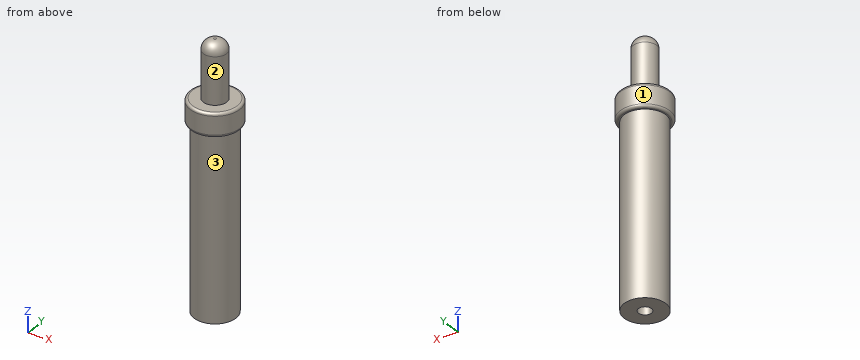
```python
from build123d import *

# Parameters (mm, degrees)
ESBO_O1_R                     = 4.7625
RESSALTO_EXTRUS_O1_DEPTH      = 50.5
FURO_ROSCADO_DE_M3X0_52_D     = 2.5
FURO_ROSCADO_DE_M3X0_52_DEPTH = 8.5
FURO_ROSCADO_DE_M3X0_52_TIP   = 0.751075774
ESBO_O8_OUTSIDE_W             = 21.979
ESBO_O8_OUTSIDE_H             = 21.979
ESBO_O8_OUTSIDE_R             = 4
CORTE_EXTRUS_O1_DEPTH         = 35
ESBO_O10_OUTSIDE_W            = 21.979
ESBO_O10_OUTSIDE_H            = 21.979
ESBO_O10_OUTSIDE_R            = 2.25
CORTE_EXTRUS_O2_DEPTH         = 11
FILETE1_R                     = 0.5
FILETE2_R                     = 2


with BuildPart() as part:
    # Esboço1 → Ressalto-extrusão1 (new body)
    with BuildSketch(Plane.XY):
        with Locations((240.708388302, 2.596082859)):
            Circle(ESBO_O1_R)
    extrude(amount=RESSALTO_EXTRUS_O1_DEPTH)

    # Furo roscado de M3x0.52
    with Locations(Plane(origin=(0, 0, 0), x_dir=(-1, 0, 0), z_dir=(0, 0, -1))):
        with Locations((-240.708388302, 2.596082859)):
            Hole(FURO_ROSCADO_DE_M3X0_52_D / 2, depth=FURO_ROSCADO_DE_M3X0_52_DEPTH)
            with Locations((0, 0, -(FURO_ROSCADO_DE_M3X0_52_DEPTH + FURO_ROSCADO_DE_M3X0_52_TIP / 2))):  # 118° drill point
                Cone(0, FURO_ROSCADO_DE_M3X0_52_D / 2, FURO_ROSCADO_DE_M3X0_52_TIP, mode=Mode.SUBTRACT)

    # Esboço8 outside → Corte-extrusão1 (cut)
    with BuildSketch(Plane(origin=(0, 0, 0), x_dir=(-1, 0, 0), z_dir=(0, 0, -1))):
        with Locations((-240.7085, 2.5965)):
            Rectangle(ESBO_O8_OUTSIDE_W, ESBO_O8_OUTSIDE_H)
        with Locations((-240.708388302, 2.596082859)):
            Circle(ESBO_O8_OUTSIDE_R, mode=Mode.SUBTRACT)
    extrude(amount=-CORTE_EXTRUS_O1_DEPTH, mode=Mode.SUBTRACT)

    # Esboço10 outside → Corte-extrusão2 (cut)
    with BuildSketch(Plane.XY.offset(50.5)):
        with Locations((240.7085, 2.5965)):
            Rectangle(ESBO_O10_OUTSIDE_W, ESBO_O10_OUTSIDE_H)
        with Locations((240.708388302, 2.596082859)):
            Circle(ESBO_O10_OUTSIDE_R, mode=Mode.SUBTRACT)
    extrude(amount=-CORTE_EXTRUS_O2_DEPTH, mode=Mode.SUBTRACT)

    # Filete1
    filete1_edges = [part.edges().sort_by_distance(p)[0] for p in [
        (235.945888302, 2.596082859, 35),
        (235.945888302, 2.596082859, 39.5),
    ]]
    fillet(filete1_edges, radius=FILETE1_R)

    # Filete2
    filete2_edges = [part.edges().sort_by_distance(p)[0] for p in [
        (238.458388302, 2.596082859, 50.5),
    ]]
    fillet(filete2_edges, radius=FILETE2_R)


solid = part.part
```
Geometry: final body of the model. Coordinates: model frame, mm. Face numbers are marked on the shaded views. A direction names the side the tool comes from. Coordinates: 2 decimals unless noted, no trailing zeros. Loops run counter-clockwise (first coordinate to the right, second up) from the corner with the lowest first, then second, coordinate; pieces in that order, holes last. Notation, with made-up numbers: (57, 48) -> (92, 48) arc R12 ccw to (92, 55) -> close; hole circle Ø10 at (70, 21.25). An arc over 180 degrees is marked (long way). Use a Markdown table: item, result. Add a question column.
(1) Pin query (flat end, axial travel): pin 1 Ø1 at (y, z) = (4.5, 27) entering from +X; pin 2 Ø3 at (y, z) = (1.5, 26) entering from -X; pin 3 Ø1 at (y, z) = (-1, 40.5) entering from +X; pin 4 Ø1.5 at (x, z) = (243, 23.5) entering from +Y. Return the tip coordinate at first contact, or that it passes through.
(2) Line query: line 1 along Z through (x, y) = (240, 5.5); line 2 along Y through (x, z) = (240.75, 9); line 3 along Z through (x, y) = (240.25, -1.5). Output: solid intervals per line, ascending.
(3) Access query for the marked faces 1, 2 and 3. Directions: +Z, -Z, +X, -X, +Y, -Y. A direction counts if a zero-diameter tool reaches every point of the face in a straight line with its end or side. Return the directions, or none.
(4) Section query A-A, the plane z = 8. Return loops of the section in (x, y).
(5) Section query B-B, the plane z = 47.5. Return loops of the section in (x, y), plus the area to 3 significant figures.
(6) Section query C-C, the plane z = 36. Return loops of the section in (x, y) (1 decimal).
Answer:
| question | item | result |
|---|---|---|
| 1 | pin 1 | stops at x = 244.45 |
| 1 | pin 2 | stops at x = 236.71 |
| 1 | pin 3 | passes through |
| 1 | pin 4 | stops at y = 6.29 |
| 2 | line 1 | z = 0 to 39.5 |
| 2 | line 2 | y = -1.4 to 2.18, 3.01 to 6.6 |
| 2 | line 3 | z = 35 to 39.5 |
| 3 | face 1 | +Z, -Z |
| 3 | face 2 | +Z |
| 3 | face 3 | -Z |
| 4 | outline | circle Ø8 at (240.71, 2.6); hole circle Ø2.5 at (240.71, 2.6) |
| 5 | outline | circle Ø4.5 at (240.71, 2.6) |
| 5 | area | 15.9 mm^2 |
| 6 | outline | circle Ø9.5 at (240.7, 2.6) |
